Check sheet for the drawn part. Datum: minimum x, y, z corner. Units: mm. A direction names the side the tool comes from. Coordinates: 2 decimals unless noted, no trailing zeros. Order: outer loops, then holes, each group sorted by start corner. A loop starts at its lowest first (then second) coordinate and runs counter-clockwise, first axis right, second up. Notation, with made-up numbers: M 25.5,-11.75 L 41.5,-11.75 A18 ccw 41.5,6.25 Z; hole C 37.5,33 d9. An arc over 180 degrees is marked long. Return JSON: item names as keys, results as strings. Group by question number.
Q1. Section check A-A, the plane x = 21. Enter the section's corners in (y, z), then the cut area to 3 significant figures.
Q2. Go/stop test with a flat-tipped pin: pin 1 Ø10 at (x, y) = (9.5, 61) entering from +Z. Record where the tip stops, or that it passes through.
Q3. Section check B-B, the plane y = 67. Enter the section's corners in (x, z).
Q4. Section check C-C, the plane z = 5. Enter the section's corners in (x, y).
Q5. Access from +Z, -Z, +X, -X, +Y, -Y to the whole of each face (thin tool, end or side, straight path). Record for the marked faces 4 and 5.
Q6. Thickness scan on probe 1 along Y at (x, z) = (88.5, 26); probe 2 along X at (y, z) = (12.5, 35). Record the ranges inside material, lowest first.
Q7. Mould release check, pull along X, two halves, no side actions. Record for the marked faces 1, 2 and 3: pulls with the +X half, pulls with the -X half, needs draft (parallel to the pull), parting line crosses it, or undercut.
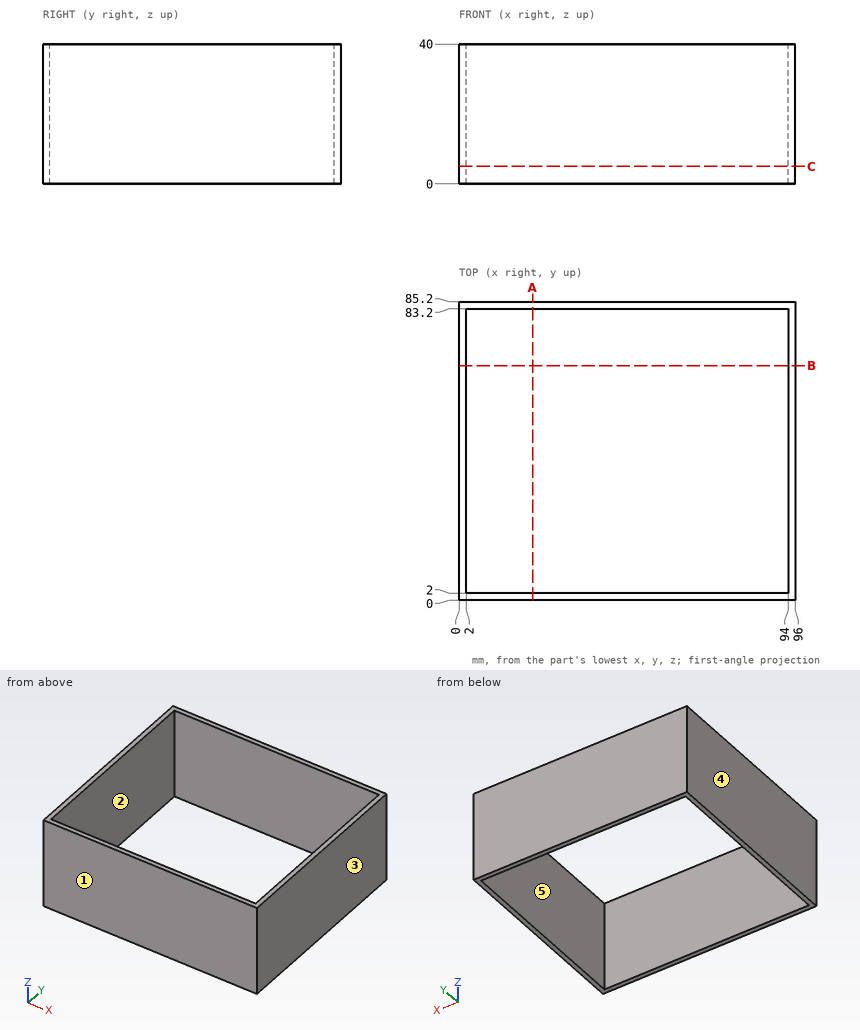
Numbers:
{
 "1": {"outline": "M 0,0 L 2,0 L 2,40 L 0,40 Z; M 83.2,0 L 85.2,0 L 85.2,40 L 83.2,40 Z", "area": "160 mm2"},
 "2": {"pin 1": "passes through"},
 "3": {"outline": "M 0,0 L 2,0 L 2,40 L 0,40 Z; M 94,0 L 96,0 L 96,40 L 94,40 Z"},
 "4": {"outline": "M 0,0 L 96,0 L 96,85.2 L 0,85.2 Z; hole M 2,2 L 94,2 L 94,83.2 L 2,83.2 Z"},
 "5": {"face 4": "+Z, -Z, -X, +Y, -Y", "face 5": "+Z, -Z"},
 "6": {"probe 1": "y = 0 to 2, 83.2 to 85.2", "probe 2": "x = 0 to 2, 94 to 96"},
 "7": {"face 1": "needs draft", "face 2": "undercut", "face 3": "pulls with the +X half"}
}
